Could you check a few things on this drawing? It's one solid part, dimensions in mm from its lowest x, y, z. A direction names the side the tool comes from. Coordinates: 2 decimals unless noted, no trailing zeros. Loops run counter-clockwise (first coordinate to the right, second up) from the corner with the lowest first, then second, coordinate; pieces in that order, holes last.
1) Imagine slicing it at D-D on z = 1.75. Please give me the cut outline in (x, y), plus the area to 3 significant figures.
2) Imagine slicing it at A-A on y = 27.5. Please give me the cut outline in (x, z), plus the area to 3 significant figures.
3) For the marked faces 1 and 2, which set-ups out of +Z, -Z, +X, -X, +Y, -Y let a thin tool reach every point of the face, with its end or its side?
4) Imagine slicing it at B-B on x = 5. Please give me the cut outline in (y, z).
5) Will these pins go through, and if not, where does the flat tip stop? P1, Ø4.5, axis at x = 50, y = 50, coming from the -Z side; P2, Ø6, axis at x = 10, y = 40.5, coming from the +Z side.
6) If I drill on line 1 along Y through (x, z) = (50, 2.6); line 2 along Z through (x, y) = (13, 43); line 3 along X through (y, z) = (16, 5.25), over which ranges is the centre line in solid material (lowest first)?
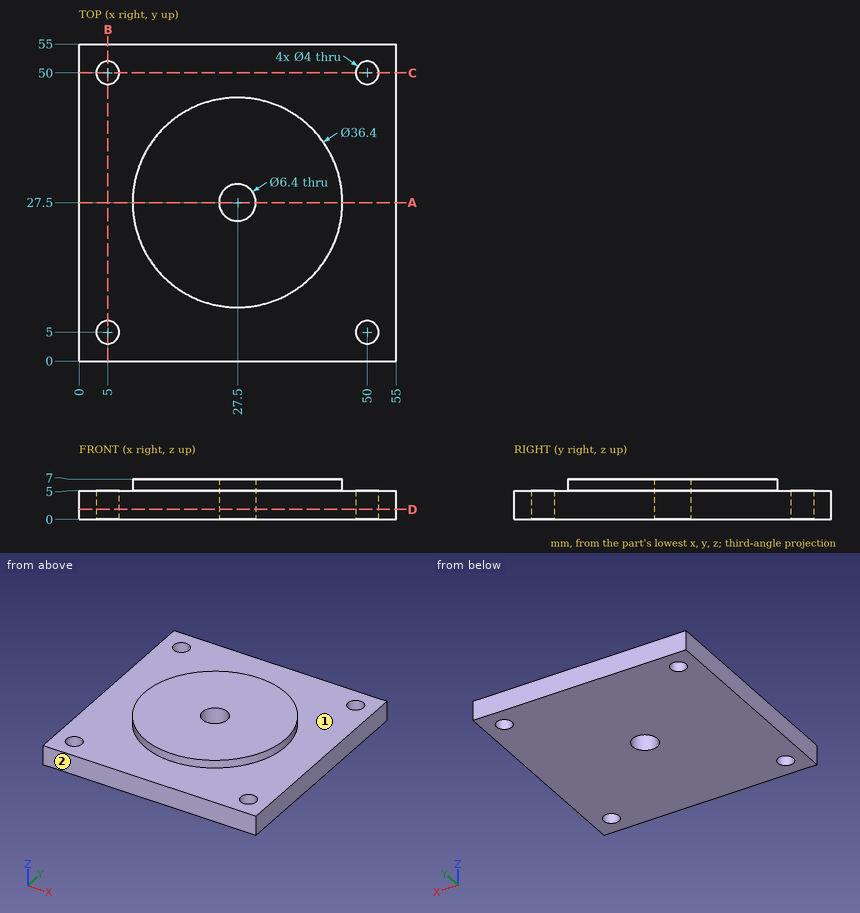
Filled in:
1. outline: (0, 0) - (55, 0) - (55, 55) - (0, 55) - close; hole circle Ø4 at (5, 5); hole circle Ø4 at (5, 50); hole circle Ø6.4 at (27.5, 27.5); hole circle Ø4 at (50, 5); hole circle Ø4 at (50, 50)
1. area: 2,940 mm2
2. outline: (0, 0) - (24.3, 0) - (24.3, 7) - (9.3, 7) - (9.3, 5) - (0, 5) - close; (30.7, 0) - (55, 0) - (55, 5) - (45.7, 5) - (45.7, 7) - (30.7, 7) - close
2. area: 303 mm2
3. face 1: +Z
3. face 2: +Z, -Z, +X, -X, -Y
4. outline: (0, 0) - (3, 0) - (3, 5) - (0, 5) - close; (7, 0) - (48, 0) - (48, 5) - (7, 5) - close; (52, 0) - (55, 0) - (55, 5) - (52, 5) - close
5. P1: stops at z = 0
5. P2: stops at z = 5
6. line 1: y = 0 to 3, 7 to 48, 52 to 55
6. line 2: z = 0 to 5
6. line 3: x = 13.39 to 41.61
